Geometry: final body of the model. Coordinates: model frame, mm. Coordinates: 2 decimals unless noted, no trailing zeros. Order: outer loops, then holes, each group sorted by start corner. A loop starts at its lowest first (then second) coordinate and runs counter-clockwise, first axis right, second up. Notation, with made-up numbers: (-30.5, 45) - (27.5, 45) arc R30 ccw to (27.5, 76) - close; hole circle Ø6 at (-4, 27.5). An arc over 180 degrees is marked (long way). Use a Markdown table: item, result. Add a question column.
```python
from build123d import *

# Parameters (mm, degrees)
BOSS_EXTRUDE1_DEPTH   = 25.4
F_6_32_TAPPED_HOLE8_D = 2.7051
CHAMFER1_SIZE         = 0.5
CHAMFER2_SIZE         = 0.5
CUT_EXTRUDE2_START    = 25.4
CUT_EXTRUDE2_DEPTH    = 10


with BuildPart() as part:
    # Sketch1 → Boss-Extrude1 (new, symmetric)
    with BuildSketch(Plane.XY):
        Polygon((3.637306696, 0), (1.818653348, 3.15), (-1.818653348, 3.15), (-3.637306696, 0), (-1.818653348, -3.15), (1.818653348, -3.15), align=None)
    extrude(amount=BOSS_EXTRUDE1_DEPTH, both=True)

    # #6-32 Tapped Hole8 (through all)
    with Locations(Plane(origin=(-0.058753338, -0.101763766, 25.4), x_dir=(1, 0, 0), z_dir=(0, 0, 1))):
        with Locations((0, 0)):
            Hole(F_6_32_TAPPED_HOLE8_D / 2)

    # Chamfer1
    chamfer1_edges = [part.edges().sort_by_distance(p)[0] for p in [
        (1.293796662, -0.101763766, 25.4),
    ]]
    chamfer(chamfer1_edges, length=CHAMFER1_SIZE)

    # Chamfer2
    chamfer2_edges = [part.edges().sort_by_distance(p)[0] for p in [
        (1.293796662, -0.101763766, -25.4),
    ]]
    chamfer(chamfer2_edges, length=CHAMFER2_SIZE)

    # Sketch1<2> → Cut-Extrude2 (cut)
    with BuildSketch(Plane.XY.offset(CUT_EXTRUDE2_START)):
        Polygon((3.637306696, 0), (1.818653348, 3.15), (-1.818653348, 3.15), (-3.637306696, 0), (-1.818653348, -3.15), (1.818653348, -3.15), align=None)
    extrude(amount=-CUT_EXTRUDE2_DEPTH, mode=Mode.SUBTRACT)


solid = part.part
```
1) Line query: line 1 (Y direction, x = -0.25, z = 1); line 2 (Y direction, x = 1, z = -12.5); line 3 (X direction, y = 0.5, z = -3). Output: solid intervals per line, ascending. Write a range as from..to.
2) Section query B-B (y = -2.5). Return the cut outline in (x, z), and give its area (3 significant figures).
3) Section query A-A (z = -17). Return the cut outline in (x, y).
4) Section query C-C (x = 2.5). Return the cut outline in (y, z).
5) Draft query along Y for faces 1 (the flat face through (2.715, -1.597, -4.714)), 2 (the flat face through (0, 3.15, -5)), 3 (the flat face through (2, 1, -25.4)), 4 (the cylindrical face through (0.94, 0.81, -5.03)). Return one class per face: released by +Y, released by -Y, zero draft, split by the parting line, or undercut.
6) First-contact query: pin 1 (3 mm diameter, centred on y = -1, z = 0, fed in from +X); pin 2 (1.5 mm diameter, centred on x = 1, y = -0.5, fed in from +Z); pin 3 (1.5 mm diameter, centred on x = 0.5, y = -1, fed in from -Z). Flat tips, straight axial feed; report the tip coordinate or a pass-through.
From the geometry:
| question | item | result |
|---|---|---|
| 1 | line 1 | y = -3.15..-1.44, 1.24..3.15 |
| 1 | line 2 | y = -3.15..-0.94, 0.74..3.15 |
| 1 | line 3 | x = -3.35..-1.27, 1.15..3.35 |
| 2 | outline | (-2.19, -25.4) - (2.19, -25.4) - (2.19, 15.4) - (-2.19, 15.4) - close |
| 2 | area | 179 mm^2 |
| 3 | outline | (-3.64, 0) - (-1.82, -3.15) - (1.82, -3.15) - (3.64, 0) - (1.82, 3.15) - (-1.82, 3.15) - close; hole circle Ø2.71 at (-0.06, -0.1) |
| 4 | outline | (-1.97, -25.4) - (1.97, -25.4) - (1.97, 15.4) - (-1.97, 15.4) - close |
| 5 | face 1 | released by -Y |
| 5 | face 2 | released by +Y |
| 5 | face 3 | zero draft |
| 5 | face 4 | undercut |
| 6 | pin 1 | stops at x = 3.64 |
| 6 | pin 2 | stops at z = 15.4 |
| 6 | pin 3 | stops at z = -25.36 |
